Read the model definition and answer for the solid it produces. Units are mm, in the model's axes. A direction names the side the tool comes from. Coordinates: 2 decimals unless noted, no trailing zeros. Write each loop counter-clockwise with the first axis right and the second up, starting at its lowest first coordinate (ties: lowest second). Pieces come first, ordered by that corner, then holes. Notation, with made-up numbers: (67.25, 49) -> (109.25, 49) arc R21 ccw to (109.25, 73) -> close; hole circle Ø9 at (26, -34). An arc over 180 degrees is marked (long way). Answer as a JSON object with one key per item and string values. Group by question number.
(1) Find section A-A (z = -2.5). Give the vertices of the cut face in (x, y).
(2) Which of the six approach directions +Z, -Z, +X, -X, +Y, -Y give full straight-line access (tool end or side, diameter ignored) to faces 1 (the face through (-2.948, 0.107, 0.542)), 2 (the face through (0.54, 2.44, 3.52))?
(3) Find section B-B (z = 1.5). Give the vertices of the cut face in (x, y).
(4) Straight lines are drawn through the part: L1, parallel to Z at x = 0.65, y = 2.6; L2, parallel to Y at x = -0.1, z = 3.5; L3, parallel to X at y = 1.15, z = -1. For each, find the intervals that lie inside material, in ascending order.
(5) Flat-ended cylindrical pins translate along their axes: P1, Ø1.5, axis at x = 0.5, z = 4.5, coming from the +Y side; P2, Ø0.6, axis at x = 0, z = -3, coming from the +Y side; P3, Ø0.6, axis at y = 1, z = -4.5, coming from the +X side. Find the tip coordinate at first contact, or state that the pin passes through.
from build123d import *

# Parameters (mm, degrees)
F3_DEPTH = 1.1
F4_W     = 0.5
F4_H     = 0.5
F5_DEPTH = 6


with BuildPart() as f1:
    # F0 (on Front) → F1 (revolve)
    with BuildSketch(Plane.XZ):
        with BuildLine():
            Line((0, 0), (0, 8.5))
            ThreePointArc((0, 8.5), (-1.767767, 7.767767), (-2.5, 6))
            Line((-2.5, 6), (-2.5, 1.1))
            Line((-2.5, 1.1), (-2.95, 1.1))
            Line((-2.95, 1.1), (-2.95, 0))
            Line((-2.95, 0), (0, 0))
        make_face()
    revolve(axis=Axis((0, 0, 11.292809), (0, 0, 1)))

    # F2 (on face) → F3 (cut, through all)
    with BuildSketch(Plane.XY.offset(1.1)):
        with BuildLine():
            Line((2.5, 1.566046), (2.5, -1.566046))
            ThreePointArc((2.5, -1.566046), (2.95, 0), (2.5, 1.566046))
        make_face()
    extrude(amount=-F3_DEPTH, mode=Mode.SUBTRACT)

    # F4 (on face) → F5 (join)
    with BuildSketch(Plane(origin=(0, 0, 0), x_dir=(1, 0, 0), z_dir=(0, 0, -1))):
        with Locations((0, 1.2)):
            Rectangle(F4_W, F4_H)
        with Locations((0, -1.2)):
            Rectangle(F4_W, F4_H)
    extrude(amount=F5_DEPTH)


solid = f1.part
Results below:
{
 "1": {"outline": "(-0.25, -1.45) -> (0.25, -1.45) -> (0.25, -0.95) -> (-0.25, -0.95) -> close; (-0.25, 0.95) -> (0.25, 0.95) -> (0.25, 1.45) -> (-0.25, 1.45) -> close"},
 "2": {"face 1": "+Z, -Z", "face 2": "+Z"},
 "3": {"outline": "circle Ø5 at (0, 0)"},
 "4": {"L1": "z = 0 to 1.1", "L2": "y = -2.5 to 2.5", "L3": "x = -0.25 to 0.25"},
 "5": {"P1": "stops at y = 2.5", "P2": "stops at y = 1.45", "P3": "stops at x = 0.25"}
}
